from build123d import *

# Parameters (mm, degrees)
F0_W     = 75
F0_H     = 75
F1_DEPTH = 5
F2_W     = 70
F2_H     = 5
F3_DEPTH = 70
F4_R     = 25
F5_R     = 2


with BuildPart() as f1:
    # F0 (on Top) → F1 (new body)
    with BuildSketch(Plane.XY):
        Rectangle(F0_W, F0_H)
    extrude(amount=F1_DEPTH)

    # F2 (on face) → F3 (join)
    with BuildSketch(Plane.XY.offset(5)):
        Polygon((-32.5, 37.5), (-37.5, 37.5), (-37.5, -37.5), (-32.5, -37.5), (-32.5, 32.5), align=None)
        with Locations((2.5, 35)):
            Rectangle(F2_W, F2_H)
    extrude(amount=F3_DEPTH)

    # F4
    f4_edges = [f1.edges().sort_by_distance(p)[0] for p in [
        (37.5, 35, 75),
        (-35, -37.5, 75),
        (37.5, -37.5, 2.5),
    ]]
    fillet(f4_edges, radius=F4_R)

    # F5
    f5_edges = [f1.edges().sort_by_distance(p)[0] for p in [
        (-12.5, -37.5, 0),
        (30.17767, -30.17767, 0),
        (-37.5, 0, 0),
        (37.5, 12.5, 0),
        (0, 37.5, 0),
        (-37.5, 12.5, 75),
        (-37.5, -30.17767, 67.67767),
        (-37.5, 37.5, 37.5),
        (-37.5, -37.5, 25),
        (37.5, 37.5, 25),
        (30.17767, 37.5, 67.67767),
        (-12.5, 37.5, 75),
    ]]
    fillet(f5_edges, radius=F5_R)


solid = f1.part
The model under review builds one solid part; all positions refer to its coordinate system, in mm. A direction names the side the tool comes from. Round coordinates to 2 decimals unless told otherwise and drop trailing zeros. Order: outer loops, then holes, each group sorted by start corner. A loop starts at its lowest first (then second) coordinate and runs counter-clockwise, first axis right, second up. Notation, with made-up numbers: (-23, 12.5) - (-5, 12.5) arc R21 ccw to (-5, 18.5) - close; hole circle Ø3 at (29.5, 23). An arc over 180 degrees is marked (long way). Use one line per item in the form item = value.
Q1. Clearance check with flat-ended pins moving along their axes: P1, Ø5, axis at y = 4, z = 38.5, coming from the +X side; P2, Ø10, axis at x = -19.5, y = -11.5, coming from the +Z side; P3, Ø3, axis at x = 6.5, z = 21, coming from the -Y side. State where each tip first meets the part, or that it passes through.
Response values:
P1 = -32.5
P2 = 5
P3 = 32.5
Q2. Tool access review of faces 1 (the flat face through (-32.5, -3, 40)), 2 (the flat face through (37.5, 22.1, 4.6)): name each direction out of +Z, -Z, +X, -X, +Y, -Y from which nothing blocks a thin tool from reaching the whole face with its end or side.
Response values:
face_1 = +Z, +X, -Y
face_2 = +Z, -Z, +X, +Y, -Y
Q3. Add section A-A on z = 46.5. Give the boundary of the cut face in (x, y).
Response values:
outline = (-37.5, -35.5) arc R2 ccw to (-35.5, -37.5) - (-32.5, -37.5) - (-32.5, 32.5) - (37.5, 32.5) - (37.5, 35.5) arc R2 ccw to (35.5, 37.5) - (-35.5, 37.5) arc R2 ccw to (-37.5, 35.5) - close
Q4. Add section B-B on x = 2. Give the boundary of the cut face in (y, z), then the cut area to 3 significant figures.
Response values:
outline = (-37.5, 2) arc R2 ccw to (-35.5, 0) - (35.5, 0) arc R2 ccw to (37.5, 2) - (37.5, 73) arc R2 ccw to (35.5, 75) - (32.5, 75) - (32.5, 5) - (-37.5, 5) - close
area = 722 mm^2
Q5. To check wall thickness, follow line 1 (Z direction, x = 9.5, y = 26.5); line 2 (Y direction, x = 18.5, z = 23); line 3 (X direction, y = -8, z = 32.5). State the ranges of each line that lie inside material, in increasing order.
Response values:
line_1 = 0 to 5
line_2 = 32.5 to 37.5
line_3 = -37.5 to -32.5
